from build123d import *

# Parameters (mm, degrees)
SKETCH1_R           = 30
SKETCH1_R_2         = 7
BOSS_EXTRUDE1_DEPTH = 10
FILLET1_R           = 10
FILLET2_R           = 20
CUT_EXTRUDE1_DEPTH  = 9
SKETCH3_R           = 9.25
SKETCH3_R_2         = 7
SKETCH3_R_3         = 5
SKETCH3_R_4         = 3.023758928
CUT_EXTRUDE2_DEPTH  = 12


with BuildPart() as part:
    # Sketch1 → Boss-Extrude1 (new body, symmetric)
    with BuildSketch(Plane.XY):
        with BuildLine():
            Line((27.935473676, 25.760615491), (128.063755469, 9.084385863))
            ThreePointArc((128.063755469, 9.084385863), (155, 0), (128.063755469, -9.084385863))
            Line((128.063755469, -9.084385863), (27.935473676, -25.760615491))
            ThreePointArc((27.935473676, -25.760615491), (-38, 0), (27.935473676, 25.760615491))
        make_face()
        Circle(SKETCH1_R, mode=Mode.SUBTRACT)
        with Locations((140, 0)):
            Circle(SKETCH1_R_2, mode=Mode.SUBTRACT)
    extrude(amount=BOSS_EXTRUDE1_DEPTH, both=True)

    # Fillet1
    fillet1_edges = [part.edges().sort_by_distance(p)[0] for p in [
        (128.063755469, 9.084385863, 0),
        (128.063755469, -9.084385863, 0),
    ]]
    fillet(fillet1_edges, radius=FILLET1_R)

    # Fillet2
    fillet2_edges = [part.edges().sort_by_distance(p)[0] for p in [
        (27.935473676, 25.760615491, 0),
        (27.935473676, -25.760615491, 0),
    ]]
    fillet(fillet2_edges, radius=FILLET2_R)

    # Sketch2 → Cut-Extrude1 (cut)
    with BuildSketch(Plane.XY.offset(10)):
        with BuildLine():
            Line((41.828554558, 17.870982725), (122.478416149, 4.438857582))
            ThreePointArc((122.478416149, 4.438857582), (126.239130435, 0), (122.478416149, -4.438857582))
            Line((122.478416149, -4.438857582), (41.828554558, -17.870982725))
            ThreePointArc((41.828554558, -17.870982725), (37.231968897, -16.217361812), (36.238855523, -11.43439331))
            ThreePointArc((36.238855523, -11.43439331), (38, 0), (36.238855523, 11.43439331))
            ThreePointArc((36.238855523, 11.43439331), (37.231968897, 16.217361812), (41.828554558, 17.870982725))
        make_face()
    cut_extrude1 = extrude(amount=-CUT_EXTRUDE1_DEPTH, mode=Mode.SUBTRACT)

    # Mirror1: Cut-Extrude1 across plane
    add(cut_extrude1.mirror(Plane.XY), mode=Mode.SUBTRACT)

    # Sketch3 → Cut-Extrude2 (cut, through all)
    with BuildSketch(Plane.XY.offset(1)):
        with Locations((50.371368822, 0)):
            Circle(SKETCH3_R)
        with Locations((74.88991016, 0)):
            Circle(SKETCH3_R_2)
        with Locations((96.440508127, 0)):
            Circle(SKETCH3_R_3)
        with Locations((112.976627131, 0)):
            Circle(SKETCH3_R_4)
    extrude(amount=-CUT_EXTRUDE2_DEPTH, mode=Mode.SUBTRACT)


solid = part.part
Design review of the part built by this model. Coordinates are the model's own, in mm. A direction names the side the tool comes from. Round coordinates to 2 decimals unless told otherwise and drop trailing zeros. Loops run counter-clockwise (first coordinate to the right, second up) from the corner with the lowest first, then second, coordinate; pieces in that order, holes last. Notation, with made-up numbers: (-5.75, 5) - (26.25, 5) arc R20 ccw to (26.25, 22) - close; hole circle Ø11 at (6.25, -25). An arc over 180 degrees is marked (long way). One line per item, written item: value. Start each with the question number.
1) Insertion check: pin 1 Ø3 at (x, z) = (89.5, 6.5) entering from -Y; pin 2 Ø1.5 at (y, z) = (30, 1.5) entering from +X; pin 3 Ø1 at (x, z) = (-16.5, 0) entering from -Y; pin 4 Ø12 at (x, y) = (65.5, 25.5) entering from -Z. Each pin has a flat end and moves straight along its axis. Give the tip position at first contact, or say it passes through.
2) Consider section A-A on x = 0. Give the boundary of the cut face in (y, z), then the cut area to 3 significant figures.
3) Consider section D-D on y = 0. Give the number of separate pieces and of enclosed holes in the cut face, then the cut area to 3 significant figures.
4) For faces 1 (the cylindrical face through (37.186, 16.163, -5.563)), 2 (the flat face through (77.872, 17.444, 0.14)), 3 (the cylindrical face through (37.186, 16.163, 5.563)), 4 (the cylindrical face through (91.445, 0.22, 0.014)), list the 3-axis set-ups (+Z, -Z, +X, -X, +Y, -Y) from which the entire face can be reached by the end or side of a thin tool; tool diameter is ignored.
5) To check wall thickness, follow L1, parallel to Y at x = 140, z = 2; L2, parallel to Y at x = 113, z = 4.5; L3, parallel to Z at x = 47, y = -12. State the ranges of each line that lie inside material, in increasing order. Write a range as from..to.
6) Consider section C-C on y = 27. Give the boundary of the cut face in (x, z).
7) Consider section B-B on z = -5. Give the boundary of the cut face in (x, y).
8) Draft analysis for pull direction Y (two halves, no side actions). For faces 5 (the cylindrical face through (28.9, 26.3, 0.1)), 6 (the cylindrical face through (37.28, -16.27, -5.56)), 7 (the flat face through (79.12, -17.236, 0.14)), state which applies: +Y half, -Y half, draft (parallel to the pull), parting line (faces both ways), or undercut.
Reported:
1. pin 1: stops at y = -15.76
1. pin 2: stops at x = 24.26
1. pin 3: stops at y = -34.47
1. pin 4: stops at z = -10
2. outline: (-38, -10) - (-30, -10) - (-30, 10) - (-38, 10) - close; (30, -10) - (38, -10) - (38, 10) - (30, 10) - close
2. area: 320 mm^2
3. separate pieces: 7
3. enclosed holes: 0
3. area: 695 mm^2
4. face 1: -Z
4. face 2: +Z, -Z, +Y
4. face 3: +Z
4. face 4: +Z, -Z
5. L1: y = -15..-7, 7..15
5. L2: y = -11.59..-6.02, 6.02..11.59
5. L3: z = -1..1
6. outline: (-26.74, -10) - (-13.08, -10) - (-13.08, 10) - (-26.74, 10) - close; (13.08, -10) - (27.51, -10) - (27.51, 10) - (13.08, 10) - close
7. outline: (24.38, -29.15) arc R20 cw to (33.92, -24.76) - (123.07, -9.92) arc R10 cw to (130.83, -11.87) arc R15 ccw (long way) to (130.83, 11.87) arc R10 cw to (123.07, 9.92) - (33.92, 24.76) arc R20 cw to (24.38, 29.15) arc R38 ccw (long way) to start; hole circle Ø60 at (0, 0); hole (36.24, -11.43) arc R5 ccw to (41.83, -17.87) - (122.48, -4.44) arc R4.5 ccw to (122.48, 4.44) - (41.83, 17.87) arc R5 ccw to (36.24, 11.43) arc R38 cw to start; hole circle Ø14 at (140, 0)
8. face 5: +Y half
8. face 6: undercut
8. face 7: -Y half
